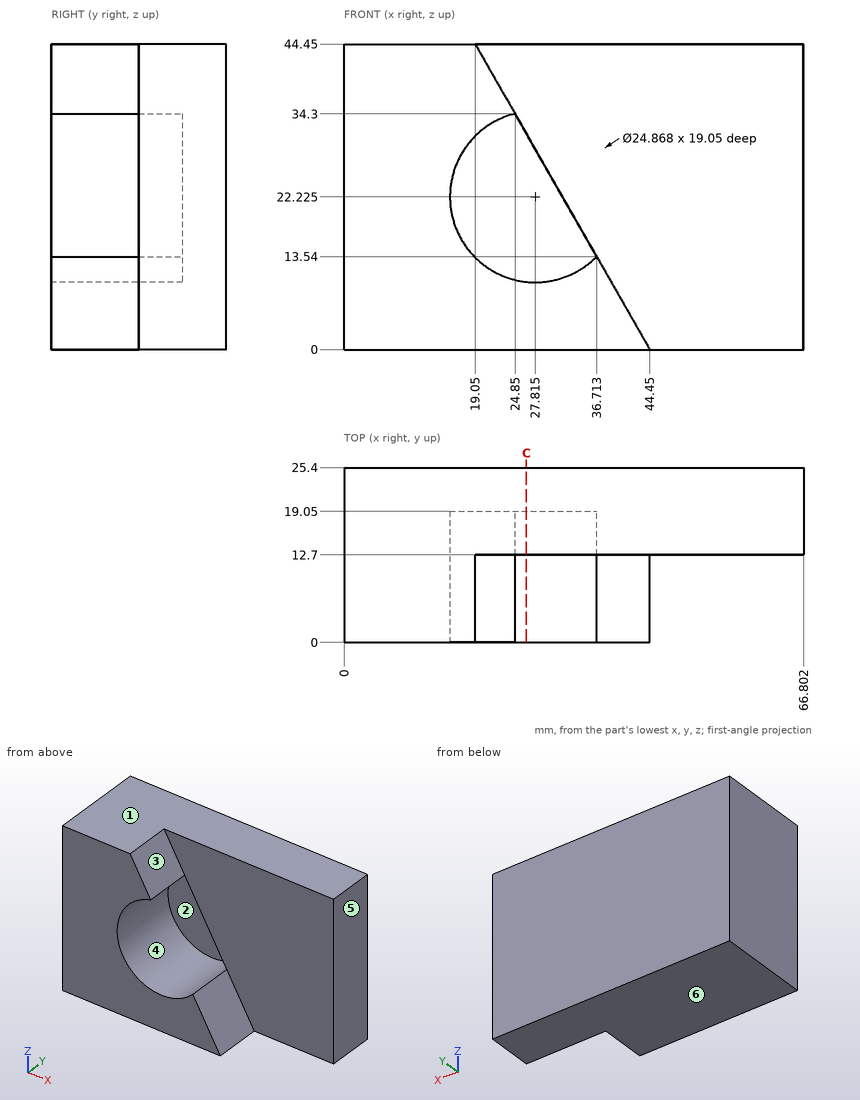
Verification items for this drawing (mm, ordinates from the low corner). A direction names the side the tool comes from. Round coordinates to 2 decimals unless told otherwise and drop trailing zeros. Loops run counter-clockwise (first coordinate to the right, second up) from the corner with the lowest first, then second, coordinate; pieces in that order, holes last. Notation, with made-up numbers: M -40,70 L 2,70 A32 cw 2,97 Z; hole C -5,-31 d7. An arc over 180 degrees is marked long. Answer as a JSON object with one key per item and string values.
1. Gauge pin test, flat ends, axial feed: P1, Ø1.5, axis at y = 7, z = 34.5, coming from the +X side; P2, Ø8, axis at x = 24, y = 5.5, coming from the +Z side (1 decimal); P3, Ø17, axis at x = 25, z = 23.5, coming from the -Y side. Record the tip position at first contact, or that the pin passes through.
Reply:
{"P1": "stops at x = 24.85", "P2": "stops at z = 42.8", "P3": "stops at y = 12.7"}
2. Access from +Z, -Z, +X, -X, +Y, -Y to the whole of each face (thin tool, end or side, straight path). Record for the marked faces 1, 2 and 3.
Reply:
{"face 1": "+Z, +X, -X, +Y, -Y", "face 2": "-Y", "face 3": "+Z, +X, -Y"}
3. Section check C-C (x = 26.5). Record the boundary of the cut face in (y, z), plus the area to 3 significant figures.
Reply:
{"outline": "M 0,0 L 25.4,0 L 25.4,44.45 L 12.7,44.45 L 12.7,31.41 L 19.05,31.41 L 19.05,9.86 L 0,9.86 Z", "area": "553 mm²"}
4. Scan lines: line 1 (Y direction, x = 29, z = 32); line 2 (Y direction, x = 28, z = 26); line 3 (X direction, y = 17.75, z = 32.5) (1 decimal). Record each from-to range of solid material in increasing order.
Reply:
{"line 1": "y = 12.7 to 25.4", "line 2": "y = 19.05 to 25.4", "line 3": "x = 0 to 20.8, 25.9 to 66.8"}
5. Mould release check, pull along X, two halves, no side actions. Record for the marked faces 4, 5 and 6: pulls with the +X half, pulls with the -X half, needs draft (parallel to the pull), parting line crosses it, or undercut.
Reply:
{"face 4": "undercut", "face 5": "pulls with the +X half", "face 6": "needs draft"}
